```python
from build123d import *

# Parameters (mm, degrees)
BOSS_EXTRUDE2_DEPTH     = 1.587
SKETCH5_R               = 2.06268814
SKETCH5_R_2             = 1.20109573
SKETCH5_R_3             = 1.525
SKETCH5_R_4             = 0.3
CUT_EXTRUDE3_DEPTH      = 49.333526863
CUT_EXTRUDE4_DEPTH      = 49.333526863
CUT_EXTRUDE5_DEPTH      = 49.333526863
CUT_EXTRUDE7_DEPTH      = 49.333526863
CUT_EXTRUDE8_DEPTH      = 49.333526863
CUT_EXTRUDE9_DEPTH      = 49.333526863
CUT_EXTRUDE9_DEPTH_BACK = 49.333526863
SKETCH6_R               = 1.625
SKETCH6_R_2             = 1.375
CUT_EXTRUDE10_DEPTH     = 49.333526863
SKETCH18_R              = 0.2921
CUT_EXTRUDE11_DEPTH     = 49.333526863


with BuildPart() as part:
    # Sketch3 → Boss-Extrude2 (new body)
    with BuildSketch(Plane(origin=(0, 0, 0), x_dir=(1, 0, 0), z_dir=(0, 1, 0))):
        with BuildLine():
            Line((-38.533712153, -25.825), (38.533712153, -25.825))
            ThreePointArc((38.533712153, -25.825), (39.08143471, -25.661660027), (39.450227292, -25.225))
            ThreePointArc((39.450227292, -25.225), (39.764339828, -24.764339828), (40.225, -24.450227292))
            ThreePointArc((40.225, -24.450227292), (40.661660027, -24.08143471), (40.825, -23.533712153))
            Line((40.825, -23.533712153), (40.825, 23.533712153))
            ThreePointArc((40.825, 23.533712153), (40.661660027, 24.08143471), (40.225, 24.450227292))
            ThreePointArc((40.225, 24.450227292), (39.764339828, 24.764339828), (39.450227292, 25.225))
            ThreePointArc((39.450227292, 25.225), (39.08143471, 25.661660027), (38.533712153, 25.825))
            Line((38.533712153, 25.825), (-38.533712153, 25.825))
            ThreePointArc((-38.533712153, 25.825), (-39.08143471, 25.661660027), (-39.450227292, 25.225))
            ThreePointArc((-39.450227292, 25.225), (-39.764339828, 24.764339828), (-40.225, 24.450227292))
            ThreePointArc((-40.225, 24.450227292), (-40.661660027, 24.08143471), (-40.825, 23.533712153))
            Line((-40.825, 23.533712153), (-40.825, -23.533712153))
            ThreePointArc((-40.825, -23.533712153), (-40.661660027, -24.08143471), (-40.225, -24.450227292))
            ThreePointArc((-40.225, -24.450227292), (-39.764339828, -24.764339828), (-39.450227292, -25.225))
            ThreePointArc((-39.450227292, -25.225), (-39.08143471, -25.661660027), (-38.533712153, -25.825))
        make_face()
    extrude(amount=BOSS_EXTRUDE2_DEPTH)

    # Sketch5 → Cut-Extrude3 (cut, through all)
    with BuildSketch(Plane(origin=(0, 0, 0), x_dir=(1, 0, 0), z_dir=(0, 1, 0))):
        with Locations(Location((30.3434, -16.665, 0), (0, 0, 270))):
            Circle(SKETCH5_R)
        with Locations(Location((22.9734, -14.125, 0), (0, 0, 270))):
            Circle(SKETCH5_R_2)
        with Locations(Location((16.6234, -14.125, 0), (0, 0, 270))):
            Circle(SKETCH5_R_2)
        with Locations(Location((10.2734, -14.125, 0), (0, 0, 270))):
            Circle(SKETCH5_R_2)
        with Locations(Location((3.9234, -14.125, 0), (0, 0, 270))):
            Circle(SKETCH5_R_2)
        with Locations(Location((-3.4466, -16.665, 0), (0, 0, 270))):
            Circle(SKETCH5_R)
        with Locations(Location((-27.825419843, 21.8, 0), (0, 0, 270))):
            Circle(SKETCH5_R_3)
        with Locations(Location((-27.825419843, -1.8, 0), (0, 0, 270))):
            Circle(SKETCH5_R_3)
        with Locations(Location((-25.057419843, 15.8, 0), (0, 0, 270))):
            Circle(SKETCH5_R_4)
        with Locations(Location((-25.057419843, 4.2, 0), (0, 0, 270))):
            Circle(SKETCH5_R_4)
    extrude(amount=CUT_EXTRUDE3_DEPTH, mode=Mode.SUBTRACT)

    # Sketch8 → Cut-Extrude4 (cut, through all)
    with BuildSketch(Plane(origin=(0, 1.587, 0), x_dir=(1, 0, 0), z_dir=(0, 1, 0))):
        with BuildLine():
            Line((4.544580157, 25.825), (4.544580157, 22.32))
            ThreePointArc((4.544580157, 22.32), (8.294580157, 18.57), (12.044580157, 22.32))
            Line((12.044580157, 22.32), (12.044580157, 25.825))
            Line((12.044580157, 25.825), (4.544580157, 25.825))
        make_face()
    extrude(amount=-CUT_EXTRUDE4_DEPTH, mode=Mode.SUBTRACT)

    # Sketch9 → Cut-Extrude5 (cut, through all)
    with BuildSketch(Plane(origin=(0, 1.587, 0), x_dir=(1, 0, 0), z_dir=(0, 1, 0))):
        with BuildLine():
            Line((-40.825, -19.825), (-34.825, -19.825))
            ThreePointArc((-34.825, -19.825), (-33.410786438, -19.239213562), (-32.825, -17.825))
            Line((-32.825, -17.825), (-32.825, -9.825))
            ThreePointArc((-32.825, -9.825), (-33.410786438, -8.410786438), (-34.825, -7.825))
            Line((-34.825, -7.825), (-40.825, -7.825))
            Line((-40.825, -7.825), (-40.825, -19.825))
        make_face()
    extrude(amount=-CUT_EXTRUDE5_DEPTH, mode=Mode.SUBTRACT)

    # Sketch10 → Cut-Extrude7 (cut, through all)
    with BuildSketch(Plane(origin=(0, 1.587, 0), x_dir=(1, 0, 0), z_dir=(0, 1, 0))):
        with BuildLine():
            Line((20.165, 23.705), (20.165, 26.825))
            Line((20.165, 26.825), (27.405, 26.825))
            Line((27.405, 26.825), (27.405, 23.705))
            ThreePointArc((27.405, 23.705), (26.344726548, 21.145273452), (23.785, 20.085))
            ThreePointArc((23.785, 20.085), (21.225273452, 21.145273452), (20.165, 23.705))
        make_face()
    extrude(amount=-CUT_EXTRUDE7_DEPTH, mode=Mode.SUBTRACT)

    # Sketch12 → Cut-Extrude8 (cut, through all)
    with BuildSketch(Plane(origin=(0, 1.587, 0), x_dir=(1, 0, 0), z_dir=(0, 1, 0))):
        with BuildLine():
            Line((-12.54393673, -26.825), (-5.30393673, -26.825))
            Line((-5.30393673, -26.825), (-5.30393673, -23.705))
            ThreePointArc((-5.30393673, -23.705), (-8.92393673, -20.085), (-12.54393673, -23.705))
            Line((-12.54393673, -23.705), (-12.54393673, -26.825))
        make_face()
    extrude(amount=-CUT_EXTRUDE8_DEPTH, mode=Mode.SUBTRACT)

    # Sketch14 → Cut-Extrude9 (cut, two sides: drawn at the far end of the back side and taken through both)
    with BuildSketch(Plane(origin=(0, 1.587, 0), x_dir=(1, 0, 0), z_dir=(0, 1, 0)).offset(-CUT_EXTRUDE9_DEPTH_BACK)):
        with BuildLine():
            Line((232.361167195, 9.825), (40.825, 9.825))
            ThreePointArc((40.825, 9.825), (38.825, 11.825), (40.825, 13.825))
            Line((40.825, 13.825), (232.361167195, 13.825))
            Line((232.361167195, 13.825), (615.433501586, 13.825))
            Line((615.433501586, 13.825), (615.433501586, 9.825))
            Line((615.433501586, 9.825), (232.361167195, 9.825))
        make_face()
    extrude(amount=CUT_EXTRUDE9_DEPTH + CUT_EXTRUDE9_DEPTH_BACK, mode=Mode.SUBTRACT)

    # Sketch6 → Cut-Extrude10 (cut, through all)
    with BuildSketch(Plane(origin=(0, 1.587, 0), x_dir=(1, 0, 0), z_dir=(0, 1, 0))):
        with Locations(Location((31.75, 16.325, 0), (0, 0, 270))):
            Circle(SKETCH6_R)
        with Locations(Location((31.75, 22.325, 0), (0, 0, 270))):
            Circle(SKETCH6_R_2)
        with Locations(Location((36.477344643, 19.375, 0), (0, 0, 270))):
            Circle(SKETCH6_R_2)
    extrude(amount=-CUT_EXTRUDE10_DEPTH, mode=Mode.SUBTRACT)

    # Sketch18 → Cut-Extrude11 (cut, through all)
    with BuildSketch(Plane(origin=(0, 1.587, 0), x_dir=(1, 0, 0), z_dir=(0, 1, 0))):
        with Locations(Location((32.968, 2.032, 0), (0, 0, 270))):
            Circle(SKETCH18_R)
        with Locations(Location((37.032, -2.032, 0), (0, 0, 270))):
            Circle(SKETCH18_R)
    extrude(amount=-CUT_EXTRUDE11_DEPTH, mode=Mode.SUBTRACT)


solid = part.part
```
Geometry: final body of the model. Coordinates: model frame, mm. A direction names the side the tool comes from. Give positions to 0.01 mm unless a question says otherwise; leave off trailing zeros. Write each loop counter-clockwise with the first axis right and the second up, starting at its lowest first coordinate (ties: lowest second). Pieces come first, ordered by that corner, then holes.
1. Section query B-B, the plane y = 1.15. Count the separate pieces of the cut face and the enclosed holes in it, then the cut area to 3 significant figures.
2. Pin query (flat end, axial travel): P1, Ø2.5, axis at x = -27.83, z = 1.8, coming from the +Y side; P2, Ø0.8, axis at y = 0.5, z = -25, coming from the -X side; P3, Ø0.8, axis at y = 1, z = 24.5, coming from the +X side; P4, Ø0.5, axis at y = 0.5, z = -24.5, coming from the +X side. Return the tip coordinate at first contact, or that it passes through.
3. Section query A-A, the plane x = -7.5. Return loops of the section in (y, z) (3 decimals), then the cut area to 3 significant figures.
4. Draft query along X for faces 1 (the cylindrical face through (21.8, 0.78, 13.86)), 2 (the flat face through (40.825, 1, -19)), 3 (the cylindrical face through (-33.426, 0.805, 19.255)). Return one class per face: released by +X, released by -X, zero draft, split by the parting line, or undercut.
5. Line query: probe 1 along X at (y, z) = (1.35, 16.5) (3 decimals); probe 2 along X at (y, z) = (0.15, -21.5) (3 decimals); probe 3 along X at (y, z) = (1.25, 1.8) (3 decimals). Output: solid intervals per line, ascending.
6. Reachability of faces 4 (the flat face through (4.545, 1, -24)), 5 (the cylindrical face through (-3.356, 0.782, 14.604)), 6 (the flat face through (-12.544, 1, 25)), 7 (the flat face through (-32.825, 1, 14)) from +Z, -Z, +X, -X, +Y, -Y: full face, straight path, thin tool, end or side. Return the list, or none.
Computed:
1. separate pieces: 1
1. enclosed holes: 15
1. area: 3,910 mm2
2. P1: passes through
2. P2: stops at x = -39.96
2. P3: stops at x = 40.65
2. P4: stops at x = 40.52
3. outline: (0, -25.825) - (1.587, -25.825) - (1.587, 20.377) - (0, 20.377) - close
3. area: 73.3 mm2
4. face 1: undercut
4. face 2: released by +X
4. face 3: released by -X
5. probe 1: x = -32.825 to -5.503, -1.391 to 28.287, 32.399 to 40.825
5. probe 2: x = -40.825 to -29.321, -26.33 to 4.635, 11.954 to 20.914, 26.656 to 30.65, 32.85 to 40.825
5. probe 3: x = -40.825 to -29.35, -26.3 to 36.855, 37.209 to 40.825
6. face 4: -Z, +Y, -Y
6. face 5: +Y, -Y
6. face 6: +Z, +Y, -Y
6. face 7: -X, +Y, -Y
